Here's how the part is built. I have some questions about the finished solid (model axes, mm). A direction names the side the tool comes from. Round coordinates to 2 decimals unless told otherwise and drop trailing zeros. Loops run counter-clockwise (first coordinate to the right, second up) from the corner with the lowest first, then second, coordinate; pieces in that order, holes last. Notation, with made-up numbers: M 89,-17.5 L 97,-17.5 A14 cw 97,7.5 Z; hole C -37.5,58 d2. An arc over 180 degrees is marked long. Answer as CSV lines item,"result".
Autodesk Inventor part; units mm, degrees
ref_plane "Work Plane1" through (0, 68, 0) normal (0, 1, 0) x (-1, 0, 0)
ref_plane "Work Plane2" through (0, 65, 0) normal (0, -1, 0) x (1, 0, 0)
ref_plane "YZ Plane" through (0, 0, 0) normal (1, 0, 0) x (0, 1, 0)
sketch "Sketch1" plane through (0, 0, 0) normal (0, 1, 0) x (-1, 0, 0)
  circle A0 centre (0, 0) radius 25
  circle A1 centre (0, -30) radius 5
  circle A2 centre (30, 0) radius 5
  circle A3 centre (0, 30) radius 5
  circle A4 centre (-30, 0) radius 5
  dimension "d0" = 50
  dimension "d1" = 10
  dimension "d2" = 30
  dimension "d5" = 360
extrude "Extrusion1" add sketch "Sketch1" along normal blind 10 contours A0
thread "Thread1"
thread "Thread2"
thread "Thread3"
thread "Thread4"
sketch "Sketch2" plane through (0, 10, 0) normal (0, 1, 0) x (1, 0, 0)
  circle A0 centre (0, 0) radius 17.5
  dimension "d17" = 35
extrude "Extrusion2" add sketch "Sketch2" along normal blind 60
sketch "Sketch3" plane through (0, 70, 0) normal (0, 1, 0) x (1, 0, 0)
  circle A0 centre (0, 0) radius 10
  dimension "d20" = 20
hole "Hole1" at (0, 70, 0) direction (0, -1, 0) diameter 8 end through all
ref_plane "Work Plane1" through (0, 68, 0) normal (0, 1, 0) x (-1, 0, 0)
ref_plane "Work Plane2" through (0, 65, 0) normal (0, -1, 0) x (1, 0, 0)
sketch "Sketch6" plane through (0, 65, 0) normal (0, -1, 0) x (1, 0, 0)
  point P0 (0, 0)
fillet "Fillet2" radius 2.5 1 edges at (-17.5, 70, 0)
thread "Thread10"
sketch "Sketch9" plane through (0, 70, 0) normal (0, 1, 0) x (1, 0, 0)
  circle A0 centre (0, 0) radius 4
  circle A1 centre (0, 0) radius 7.5
  dimension "d61" = 15
hole "Hole3" at (0, 70, 0) direction (0, -1, 0) diameter 15 depth 15 tip angle 118
thread "Thread11"
sketch "Sketch10" plane through (0, 0, 0) normal (0, -1, 0) x (1, 0, 0)
  circle A0 centre (-21, 0) radius 2.75
  circle A1 centre (-10.5, -18.1865) radius 2.75
  circle A2 centre (10.5, -18.1865) radius 2.75
  circle A3 centre (21, 0) radius 2.75
  circle A4 centre (10.5, 18.1865) radius 2.75
  circle A5 centre (-10.5, 18.1865) radius 2.75
  point P0 (0, 0)
  dimension "d71" = 5.5
  dimension "d72" = 21
  dimension "d75" = 360
hole "Hole4" at (-21, 0, 0) at (-10.5, 0, 18.1865) at (10.5, 0, 18.1865) at (21, 0, 0) at (10.5, 0, -18.1865) at (-10.5, 0, -18.1865) direction (0, 1, 0) diameter 5 depth 10 tip angle 118
thread "Thread12"
thread "Thread13"
thread "Thread14"
thread "Thread15"
thread "Thread16"
thread "Thread17"
properties part number "pintle body" material "Aluminum 6061"
1. I want a section at A-A, the plane z = 0. Please give me the cut outline in (x, y), and give its area (3 significant figures).
Evaluation:
outline,"M -25,0 L -23.5,0 L -23.5,10 L -25,10 Z; M -18.5,0 L -4,0 L -4,52.9 L -7.5,55 L -7.5,70 L -15,70 A2.5 ccw -17.5,67.5 L -17.5,10 L -18.5,10 Z; M 4,0 L 18.5,0 L 18.5,10 L 17.5,10 L 17.5,67.5 A2.5 ccw 15,70 L 7.5,70 L 7.5,55 L 4,52.9 Z; M 23.5,0 L 25,0 L 25,10 L 23.5,10 Z"
area,"1,820 mm²"
2. I want a section at B-B, the plane y = 35.5. Please give me the cut outline in (x, z).
Evaluation:
outline,"C 0,0 d35; hole C 0,0 d8"
3. Which directions (+Z, -Z, +X, -X, +Y, -Y) give clear straight access to the entire face, cutting with the end or side of a thin tool? Please do faces 1 (the cylindrical face through (-8.06, 5.07, -17.64)), 2 (the cylindrical face through (-0.33, 62.395, -7.493)).
Evaluation:
face 1,"+Y, -Y"
face 2,"+Y"
4. We'd pull the mould along X, two halves only. Please class faces 3 (the cylindrical face through (-9.54, 5.07, 15.88)), 4 (the cylindrical face through (-13.887, 38.348, -10.648)), 5 (the flat face through (6, 10, 17)), 6 (the cylindrical face through (3.905, 26.078, -0.867)): pulls with the +X half, pulls with the -X half, needs draft (parallel to the pull), parting line crosses it, or undercut.
Evaluation:
face 3,"undercut"
face 4,"parting line crosses it"
face 5,"needs draft"
face 6,"undercut"
5. I want a section at D-D, the plane x = 19.5. Please give me the cut outline in (y, z).
Evaluation:
outline,"M 0,-15.64 L 10,-15.64 L 10,-2 L 0,-2 Z; M 0,2 L 10,2 L 10,15.64 L 0,15.64 Z"
6. For P1, Ø6, axis at x = -19, z = 13.5, coming from the +Y side; P2, Ø4, axis at x = 10.5, z = -18.19, coming from the +Y side; P3, Ø2, axis at x = 9.5, y = 30.5, coming from the +Z side; P4, Ø1, axis at x = 3.5, y = 41.5, coming from the +Z side, each with a flat end and sliding along its axis, tell me the tip position at first contact or that it passes through.
Evaluation:
P1,"stops at y = 10"
P2,"passes through"
P3,"stops at z = 15.3"
P4,"stops at z = 17.24"
7. If I drill on line 1 (X direction, y = 6, z = 0); line 2 (X direction, y = 34, z = 0), over which ranges is the centre line in solid material (lowest first)? Write a range as [from, to].
Evaluation:
line 1,"x = [-25, -23.5], [-18.5, -4], [4, 18.5], [23.5, 25]"
line 2,"x = [-17.5, -4], [4, 17.5]"
8. I want a section at C-C, the plane z = 18.5. Please give me the cut outline in (x, y), and give its area (3 significant figures).
Evaluation:
outline,"M -16.82,0 L -12.98,0 L -12.98,10 L -16.82,10 Z; M -8.02,0 L 8.02,0 L 8.02,10 L -8.02,10 Z; M 12.98,0 L 16.82,0 L 16.82,10 L 12.98,10 Z"
area,"237 mm²"
